The listing builds one solid part. Answer for the finished solid, in the listing's coordinates (mm). A direction names the side the tool comes from. Give positions to 0.01 mm unless a question says otherwise; leave off trailing zeros. Loops run counter-clockwise (first coordinate to the right, second up) from the corner with the lowest first, then second, coordinate; pieces in that order, holes last.
Item 1: Each of these flat-tipped pins is pushed along its axis until it touches: pin 1 Ø18 at (x, y) = (5, 30) entering from -Z; pin 2 Ø6 at (y, z) = (50, 45) entering from -X; pin 3 Ø15 at (x, z) = (76.5, 6) entering from +Y. Where does it stop, or does it pass through?
Item 2: Consider line 1 along X through (y, z) = (42.5, 7); line 2 along Z through (x, y) = (0, -4.5); line 3 along X through (y, z) = (-12, -10). Determine where each line is inside the solid, lowest interval first.
Item 3: A tool of negligible diameter and unlimited length cuts with its end or side. For faces 4 (the face through (-60, 24, 12)), 5 (the face through (20, 50, 40)), 6 (the face through (1, -30, -30)), 7 (the face through (60, 24, 12)), from which of +Z, -Z, +X, -X, +Y, -Y can it reach the whole face along a straight path? Write none if from no direction.
Item 4: The mould has two halves that part along Z. Classify faces 1 (the face through (1, 17, 30)), 2 (the face through (19.98, -9.86, -9.12)), 3 (the face through (-90, -15, 1)): pulls with the +Z half, pulls with the -Z half, needs draft (parallel to the pull), parting line crosses it, or undercut.
Item 5: Section A-A, the plane y = 48 is taken. Give the vertices of the cut face in (x, z), and give its area (3 significant figures).
Item 6: Section D-D, the plane x = 27 is taken. Give the vertices of the cut face in (y, z), and give its area (3 significant figures).
Item 7: Section B-B, the plane z = -4 is taken. Give the vertices of the cut face in (x, y), and give its area (3 significant figures).
Item 8: Section C-C, the plane y = 14 is taken. Give the vertices of the cut face in (x, z), and give its area (3 significant figures).
from build123d import *

# Parameters (mm, degrees)
SKETCH2_W           = 180
SKETCH2_H           = 100
BOSS_EXTRUDE2_DEPTH = 40
BOSS_EXTRUDE3_DEPTH = 60
SKETCH7_W           = 60
SKETCH7_H           = 40
CUT_EXTRUDE1_DEPTH  = 197.214168703
SKETCH15_W          = 80
SKETCH15_H          = 60
CUT_EXTRUDE2_DEPTH  = 80
CUT_EXTRUDE3_DEPTH  = 20
SKETCH20_R          = 20
CUT_EXTRUDE5_DEPTH  = 20


with BuildPart() as part:
    # Sketch2 → Boss-Extrude2 (new body)
    with BuildSketch(Plane(origin=(0, 0, 0), x_dir=(1, 0, 0), z_dir=(0, 1, 0))):
        Rectangle(SKETCH2_W, SKETCH2_H)
    extrude(amount=-BOSS_EXTRUDE2_DEPTH)

    # Sketch6 → Boss-Extrude3 (add, symmetric)
    with BuildSketch(Plane(origin=(0, 0, 0), x_dir=(0, 0, -1), z_dir=(1, 0, 0))):
        Polygon((50, 0), (50, 20), (-10, 60), (-50, 60), (-50, 0), align=None)
    extrude(amount=BOSS_EXTRUDE3_DEPTH, both=True)

    # Sketch7 → Cut-Extrude1 (cut, through all)
    with BuildSketch(Plane(origin=(90, 0, 0), x_dir=(0, 0, -1), z_dir=(1, 0, 0))):
        with Locations((0, -40)):
            Rectangle(SKETCH7_W, SKETCH7_H)
    extrude(amount=-CUT_EXTRUDE1_DEPTH, mode=Mode.SUBTRACT)

    # Sketch15 → Cut-Extrude2 (cut)
    with BuildSketch(Plane(origin=(0, 0, -50), x_dir=(-1, 0, 0), z_dir=(0, 0, -1))):
        with Locations((0, 30)):
            Rectangle(SKETCH15_W, SKETCH15_H)
    extrude(amount=-CUT_EXTRUDE2_DEPTH, mode=Mode.SUBTRACT)

    # Sketch16 → Cut-Extrude3 (cut)
    with BuildSketch(Plane(origin=(0, 0, 30), x_dir=(-1, 0, 0), z_dir=(0, 0, -1))):
        Polygon((20, 80), (-20, 80), (-20, 60), (1.28e-07, 60), (20, 60), align=None)
        with BuildLine():
            Line((1.28e-07, 60), (-20, 60))
            Line((-20, 60), (-20, 40))
            ThreePointArc((-20, 40), (-14.142135579, 54.142135669), (1.28e-07, 60))
        make_face()
        with BuildLine():
            ThreePointArc((1.28e-07, 60), (-14.142135579, 54.142135669), (-20, 40))
            Line((-20, 40), (20, 40))
            ThreePointArc((20, 40), (14.142135669, 54.142135579), (1.28e-07, 60))
        make_face()
        with BuildLine():
            Line((20, 40), (-20, 40))
            ThreePointArc((-20, 40), (0, 20), (20, 40))
        make_face()
        with BuildLine():
            Line((20, 40), (20, 60))
            Line((20, 60), (1.28e-07, 60))
            ThreePointArc((1.28e-07, 60), (14.142135669, 54.142135579), (20, 40))
        make_face()
    extrude(amount=-CUT_EXTRUDE3_DEPTH, mode=Mode.SUBTRACT)

    # Sketch20 → Cut-Extrude5 (cut)
    with BuildSketch(Plane(origin=(0, 0, 0), x_dir=(1, 0, 0), z_dir=(0, 1, 0))):
        with Locations(Location((0, 10, 0), (0, 0, 180))):
            Circle(SKETCH20_R)
    extrude(amount=-CUT_EXTRUDE5_DEPTH, mode=Mode.SUBTRACT)


solid = part.part
Worked answers:
1. pin 1: stops at z = 30
1. pin 2: stops at x = -60
1. pin 3: stops at y = 0
2. line 1: x = -60 to -40, 40 to 60
2. line 2: z = -50 to -30, 10 to 50
2. line 3: x = -90 to -20, 20 to 90
3. face 4: +Z, -Z, -X, +Y
3. face 5: +Z, -Z, +Y
3. face 6: +X, -X, -Y
3. face 7: +Z, -Z, +X, +Y
4. face 1: pulls with the -Z half
4. face 2: undercut
4. face 3: needs draft
5. outline: (-60, -8) - (-40, -8) - (-40, 30) - (-20, 30) - (-20, 50) - (-60, 50) - close; (20, 30) - (40, 30) - (40, -8) - (60, -8) - (60, 50) - (20, 50) - close
5. area: 3,120 mm2
6. outline: (-40, -50) - (0, -50) - (0, 30) - (60, 30) - (60, 50) - (-40, 50) - (-40, 30) - (-20, 30) - (-20, -30) - (-40, -30) - close
6. area: 4,000 mm2
7. outline: (-90, -20) - (-19.08, -20) - (-19.08, 0) - (-40, 0) - (-40, 50.67) - (-60, 50.67) - (-60, 0) - (-90, 0) - close; (19.08, -20) - (90, -20) - (90, 0) - (60, 0) - (60, 50.67) - (40, 50.67) - (40, 0) - (19.08, 0) - close
7. area: 4,860 mm2
8. outline: (-60, -50) - (-40, -50) - (-40, 30) - (40, 30) - (40, -50) - (60, -50) - (60, 50) - (-60, 50) - close
8. area: 5,600 mm2
